Check sheet for the modelled part. Datum: model origin and axes. Units: mm. Face numbers are marked on the shaded views. Round coordinates to 2 decimals unless told otherwise and drop trailing zeros. Order: outer loops, then holes, each group sorted by start corner. A loop starts at its lowest first (then second) coordinate and runs counter-clockwise, first axis right, second up. Notation, with made-up numbers: (15.25, 64) -> (21.25, 64) arc R27 cw to (21.25, 93) -> close; hole circle Ø9 at (14, -28.75). An arc over 180 degrees is marked (long way). Answer in a Markdown table with one row per item. Add a question column.
1. Sectioned sample at D-D, the plane z = 12. Record the boundary of the cut face in (x, y), then the cut area to 3 significant figures.
2. Sectioned sample at A-A, the plane y = 2. Record the boundary of the cut face in (x, z), then the cut area to 3 significant figures.
3. Draft check along Z on the marked faces 1, 2 and 3. Enter one of: +Z half, -Z half, draft (parallel to the pull), parting line (faces both ways), or undercut.
4. Depth check by flat-ended pin: P1, Ø0.9, axis at y = 9.5, z = -16, coming from the +X side; P2, Ø10, axis at x = 12.5, y = 10.5, coming from the -Z side; P3, Ø1.5, axis at y = 10.5, z = -15.5, coming from the -X side. Enter the tip coordinate at first touch or a pass-through.
5. Sectioned sample at C-C, the plane x = 11.5. Record the boundary of the cut face in (y, z).
6. Material ranges on L1, parallel to X at y = 7.5, z = 0; L2, parallel to Z at x = 0, y = 6; L3, parallel to Z at x = -10, y = 6, recorded low to high. Write a range as from..to.
7. Sectioned sample at B-B, the plane x = 0. Record the boundary of the cut face in (y, z).
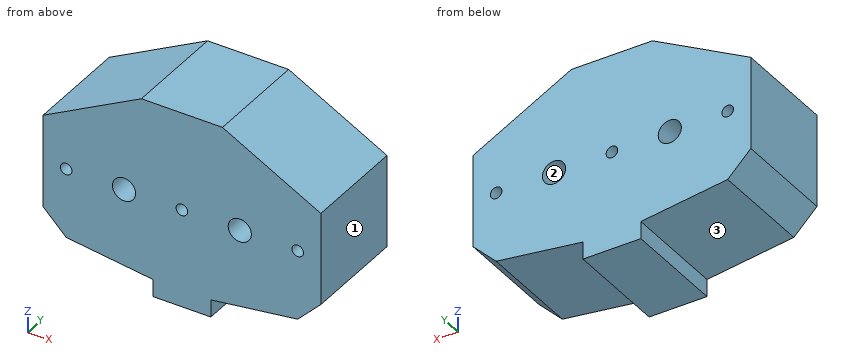
```python
from build123d import *

# Parameters (mm, degrees)
SKETCH_1_R      = 1
SKETCH_1_R_2    = 2
EXTRUDE_1_DEPTH = 18


with BuildPart() as part:
    # Эскиз1 → Бобышка-Вытянуть1 (new body)
    with BuildSketch(Plane(origin=(0, 0, 0), x_dir=(1, 0, 0), z_dir=(0, 1, 0))):
        Polygon((24, 8), (24, -8), (7, -17), (-7, -17), (-24, -8), (-24, 8), (-20, 12), (-5, 14), (-5, 17), (5, 17), (5, 14), (20, 12), align=None)
        Circle(SKETCH_1_R, mode=Mode.SUBTRACT)
        with Locations((20, 0)):
            Circle(SKETCH_1_R, mode=Mode.SUBTRACT)
        with Locations((-20, 0)):
            Circle(SKETCH_1_R, mode=Mode.SUBTRACT)
        with Locations((-10, 0)):
            Circle(SKETCH_1_R_2, mode=Mode.SUBTRACT)
        with Locations((10, 0)):
            Circle(SKETCH_1_R_2, mode=Mode.SUBTRACT)
    extrude(amount=EXTRUDE_1_DEPTH)


solid = part.part
```
Answer key:
| question | item | result |
|---|---|---|
| 1 | outline | (-16.44, 0) -> (16.44, 0) -> (16.44, 18) -> (-16.44, 18) -> close |
| 1 | area | 592 mm² |
| 2 | outline | (-24, -8) -> (-20, -12) -> (-5, -14) -> (-5, -17) -> (5, -17) -> (5, -14) -> (20, -12) -> (24, -8) -> (24, 8) -> (7, 17) -> (-7, 17) -> (-24, 8) -> close; hole circle Ø2 at (-20, 0); hole circle Ø4 at (-10, 0); hole circle Ø2 at (0, 0); hole circle Ø4 at (10, 0); hole circle Ø2 at (20, 0) |
| 2 | area | 1,270 mm² |
| 3 | face 1 | draft |
| 3 | face 2 | undercut |
| 3 | face 3 | -Z half |
| 4 | P1 | stops at x = 5 |
| 4 | P2 | stops at z = -13.67 |
| 4 | P3 | stops at x = -5 |
| 5 | outline | (0, -13.13) -> (18, -13.13) -> (18, -1.32) -> (0, -1.32) -> close; (0, 1.32) -> (18, 1.32) -> (18, 14.62) -> (0, 14.62) -> close |
| 6 | L1 | x = -24..-21, -19..-12, -8..-1, 1..8, 12..19, 21..24 |
| 6 | L2 | z = -17..-1, 1..17 |
| 6 | L3 | z = -13.33..-2, 2..15.41 |
| 7 | outline | (0, -17) -> (18, -17) -> (18, -1) -> (0, -1) -> close; (0, 1) -> (18, 1) -> (18, 17) -> (0, 17) -> close |
